```python
from build123d import *

# Parameters (mm, degrees)
SKETCH_1_W          = 150
SKETCH_1_H          = 18
EXTRUDE_1_DEPTH     = 7
CUT_EXTRUDE_1_REACH = 153.238
SKETCH_3_R          = 1.5
CUT_EXTRUDE_2_REACH = 153.238
CUT_EXTRUDE_3_REACH = 152.957
SKETCH_5_W          = 3
SKETCH_5_H          = 2.458845727
SKETCH_6_R          = 3
CUT_EXTRUDE_4_DEPTH = 3


with BuildPart() as part:
    # 草图1 → 凸台-拉伸1 (new body)
    with BuildSketch(Plane.XY):
        with Locations((75, 9)):
            Rectangle(SKETCH_1_W, SKETCH_1_H)
    extrude(amount=EXTRUDE_1_DEPTH)

    # 草图3 → 切除-拉伸1 (cut, up to next)
    with BuildSketch(Plane.XY.offset(7), mode=Mode.PRIVATE) as cut_extrude_1_sk1:
        with Locations((5, 9)):
            Circle(SKETCH_3_R)
    cut_extrude_1_tool1 = extrude(cut_extrude_1_sk1.sketch, amount=-CUT_EXTRUDE_1_REACH, mode=Mode.PRIVATE) & part.part
    # 草图3 → 切除-拉伸1 (cut, up to next)
    with BuildSketch(Plane.XY.offset(7), mode=Mode.PRIVATE) as cut_extrude_1_sk2:
        with Locations(Location((145, 9, 0), (0, 0, 180))):
            Circle(SKETCH_3_R)
    cut_extrude_1_tool2 = extrude(cut_extrude_1_sk2.sketch, amount=-CUT_EXTRUDE_1_REACH, mode=Mode.PRIVATE) & part.part
    add(cut_extrude_1_tool1.solids().sort_by_distance((5, 9, 7))[0], mode=Mode.SUBTRACT)
    add(cut_extrude_1_tool2.solids().sort_by_distance((145, 9, 7))[0], mode=Mode.SUBTRACT)

    # 草图2 → 切除-拉伸2 (cut, up to next)
    with BuildSketch(Plane(origin=(150, 0, 0), x_dir=(0, 0, -1), z_dir=(1, 0, 0)), mode=Mode.PRIVATE) as cut_extrude_2_sk1:
        Polygon((-7, 18), (-7, 13.9), (-4.9, 13.9), (-4, 15.458845727), (-3.1, 13.9), (0, 13.9), (0, 18), align=None)
    cut_extrude_2_tool1 = extrude(cut_extrude_2_sk1.sketch, amount=-CUT_EXTRUDE_2_REACH, mode=Mode.PRIVATE) & part.part
    # 草图2 → 切除-拉伸2 (cut, up to next)
    with BuildSketch(Plane(origin=(150, 0, 0), x_dir=(0, 0, -1), z_dir=(1, 0, 0)), mode=Mode.PRIVATE) as cut_extrude_2_sk2:
        Polygon((-4.9, 4.1), (-7, 4.1), (-7, 0), (0, 0), (0, 4.1), (-3.1, 4.1), (-4, 2.541154273), align=None)
    cut_extrude_2_tool2 = extrude(cut_extrude_2_sk2.sketch, amount=-CUT_EXTRUDE_2_REACH, mode=Mode.PRIVATE) & part.part
    add(cut_extrude_2_tool1.solids().sort_by_distance((150, 16.028656, 3.474302))[0], mode=Mode.SUBTRACT)
    add(cut_extrude_2_tool2.solids().sort_by_distance((150, 1.971344, 3.474302))[0], mode=Mode.SUBTRACT)

    # 草图5 → 切除-拉伸3 (cut, up to next)
    with BuildSketch(Plane.XY.offset(7), mode=Mode.PRIVATE) as cut_extrude_3_sk1:
        with Locations((1.5, 14.229422864)):
            Rectangle(SKETCH_5_W, SKETCH_5_H)
    cut_extrude_3_tool1 = extrude(cut_extrude_3_sk1.sketch, amount=-CUT_EXTRUDE_3_REACH, mode=Mode.PRIVATE) & part.part
    # 草图5 → 切除-拉伸3 (cut, up to next)
    with BuildSketch(Plane.XY.offset(7), mode=Mode.PRIVATE) as cut_extrude_3_sk2:
        with Locations((1.5, 3.770577137)):
            Rectangle(SKETCH_5_W, SKETCH_5_H)
    cut_extrude_3_tool2 = extrude(cut_extrude_3_sk2.sketch, amount=-CUT_EXTRUDE_3_REACH, mode=Mode.PRIVATE) & part.part
    # 草图5 → 切除-拉伸3 (cut, up to next)
    with BuildSketch(Plane.XY.offset(7), mode=Mode.PRIVATE) as cut_extrude_3_sk3:
        with Locations((148.5, 3.770577137)):
            Rectangle(SKETCH_5_W, SKETCH_5_H)
    cut_extrude_3_tool3 = extrude(cut_extrude_3_sk3.sketch, amount=-CUT_EXTRUDE_3_REACH, mode=Mode.PRIVATE) & part.part
    # 草图5 → 切除-拉伸3 (cut, up to next)
    with BuildSketch(Plane.XY.offset(7), mode=Mode.PRIVATE) as cut_extrude_3_sk4:
        with Locations((148.5, 14.229422864)):
            Rectangle(SKETCH_5_W, SKETCH_5_H)
    cut_extrude_3_tool4 = extrude(cut_extrude_3_sk4.sketch, amount=-CUT_EXTRUDE_3_REACH, mode=Mode.PRIVATE) & part.part
    add(cut_extrude_3_tool1.solids().sort_by_distance((1.5, 14.229423, 7))[0], mode=Mode.SUBTRACT)
    add(cut_extrude_3_tool2.solids().sort_by_distance((1.5, 3.770577, 7))[0], mode=Mode.SUBTRACT)
    add(cut_extrude_3_tool3.solids().sort_by_distance((148.5, 3.770577, 7))[0], mode=Mode.SUBTRACT)
    add(cut_extrude_3_tool4.solids().sort_by_distance((148.5, 14.229423, 7))[0], mode=Mode.SUBTRACT)

    # 草图6 → 切除-拉伸4 (cut)
    with BuildSketch(Plane(origin=(0, 0, 0), x_dir=(-1, 0, 0), z_dir=(0, 0, -1))):
        with Locations((-105, 9)):
            Circle(SKETCH_6_R)
        with Locations((-45, 9)):
            Circle(SKETCH_6_R)
    extrude(amount=-CUT_EXTRUDE_4_DEPTH, mode=Mode.SUBTRACT)


solid = part.part
```
CAD build for the part. Positions are in the model's coordinates, mm. A direction names the side the tool comes from. Round coordinates to 2 decimals unless told otherwise and drop trailing zeros. Order: outer loops, then holes, each group sorted by start corner. A loop starts at its lowest first (then second) coordinate and runs counter-clockwise, first axis right, second up.
Q1. Slice it at C-C (x = 105). Write the cut outline in (y, z), and give its area (3 significant figures).
Q2. Drop flat-ended pins along their axis: pin 1 (5 mm diameter, centred on x = 103.5, y = 10.5, fed in from -Z); pin 2 (1.7 mm diameter, centred on x = 64.5, z = 5.5, fed in from -Y); pin 3 (1.5 mm diameter, centred on x = 50.5, z = 1.5, fed in from -Y); pin 4 (0.7 mm diameter, centred on y = 3.5, z = 5, fed in from -X) (1 decimal). Give the stop position or say it passes through.
Q3. Which spindle directions (+Z, -Z, +X, -X, +Y, -Y) get a long thin tool onto all of the face, cutting with end or side? Do faces 4 (the flat face through (148, 5, 4)), 5 (the flat face through (1, 5, 4)), 6 (the cylindrical face through (107.4, 7.2, 1.5)), 7 (the flat face through (76, 4.1, 2)), 8 (the flat face through (147, 14, 4)). Say none if no direction does.
Q4. Slice it at A-A (x = 5). Write the cut outline in (y, z), and give its area (3 significant figures).
Q5. Wall check: L1, parallel to X at y = 8.75, z = 5.5; L2, parallel to X at y = 7.75, z = 2.75; L3, parallel to X at y = 7, z = 1.75. Give the ranges that are in metal, low to high.
Q6. Slice it at B-B (y = 9). Write the cut outline in (x, z).
Q7. Two-plate mould, pull along X, no slides. Class faces 1 (the flat face through (147, 4, 4)), 2 (the cylindrical face through (48, 9, 1)), 3 (the flat face through (148, 13, 4)): pulls with the +X half, pulls with the -X half, needs draft (parallel to the pull), parting line crosses it, or undercut.
Results below:
1. outline: (2.54, 4) - (4.1, 3.1) - (4.1, 0) - (6, 0) - (6, 3) - (12, 3) - (12, 0) - (13.9, 0) - (13.9, 3.1) - (15.46, 4) - (13.9, 4.9) - (13.9, 7) - (4.1, 7) - (4.1, 4.9) - close
1. area: 53.4 mm2
2. pin 1: stops at z = 0
2. pin 2: stops at y = 3.67
2. pin 3: stops at y = 4.1
2. pin 4: passes through
3. face 4: +Z, -Z, +X, -Y
3. face 5: +Z, -Z, -X, -Y
3. face 6: -Z
3. face 7: -Z, +X, -X, -Y
3. face 8: +Z, -Z, +X, +Y
4. outline: (2.54, 4) - (4.1, 3.1) - (4.1, 0) - (7.5, 0) - (7.5, 7) - (4.1, 7) - (4.1, 4.9) - close; (10.5, 0) - (13.9, 0) - (13.9, 3.1) - (15.46, 4) - (13.9, 4.9) - (13.9, 7) - (10.5, 7) - close
4. area: 50.4 mm2
5. L1: x = 0 to 3.52, 6.48 to 143.52, 146.48 to 150
5. L2: x = 0 to 4.17, 5.83 to 42.27, 47.73 to 102.27, 107.73 to 144.17, 145.83 to 150
5. L3: x = 0 to 42.76, 47.24 to 102.76, 107.24 to 150
6. outline: (0, 0) - (3.5, 0) - (3.5, 7) - (0, 7) - close; (6.5, 0) - (42, 0) - (42, 3) - (48, 3) - (48, 0) - (102, 0) - (102, 3) - (108, 3) - (108, 0) - (143.5, 0) - (143.5, 7) - (6.5, 7) - close; (146.5, 0) - (150, 0) - (150, 7) - (146.5, 7) - close
7. face 1: pulls with the +X half
7. face 2: undercut
7. face 3: needs draft
